```python
from build123d import *

# Parameters (mm, degrees)
SKETCH1_W           = 34
SKETCH1_H           = 70
BOSS_EXTRUDE1_DEPTH = 14
SKETCH2_W           = 30
SKETCH2_H           = 66
CUT_EXTRUDE1_DEPTH  = 12
SKETCH3_R           = 3
BOSS_EXTRUDE2_DEPTH = 12
SKETCH4_R           = 2
CUT_EXTRUDE2_DEPTH  = 80.069589603
CUT_EXTRUDE4_REACH  = 81.07
SKETCH6_R           = 2.5
SKETCH6_R_2         = 2
FILLET1_R           = 1
BOSS_EXTRUDE3_START = -8
SKETCH7_R           = 5
SKETCH7_R_2         = 3
BOSS_EXTRUDE3_DEPTH = 8
CUT_EXTRUDE7_START  = -4
SKETCH8_R           = 3
CUT_EXTRUDE7_DEPTH  = 4
FILLET2_R           = 2


with BuildPart() as part:
    # Sketch1 → Boss-Extrude1 (new body)
    with BuildSketch(Plane.XY):
        with Locations((17, 35)):
            Rectangle(SKETCH1_W, SKETCH1_H)
    extrude(amount=BOSS_EXTRUDE1_DEPTH)

    # Sketch2 → Cut-Extrude1 (cut)
    with BuildSketch(Plane(origin=(0, 0, 0), x_dir=(-1, 0, 0), z_dir=(0, 0, -1))):
        with Locations((-17, 35)):
            Rectangle(SKETCH2_W, SKETCH2_H)
    extrude(amount=-CUT_EXTRUDE1_DEPTH, mode=Mode.SUBTRACT)

    # Sketch3 → Boss-Extrude2 (add)
    with BuildSketch(Plane(origin=(0, 0, 0), x_dir=(-1, 0, 0), z_dir=(0, 0, -1))):
        with Locations((-31, 67)):
            Circle(SKETCH3_R)
        with Locations((-3, 67)):
            Circle(SKETCH3_R)
        with Locations((-3, 3)):
            Circle(SKETCH3_R)
        with Locations((-31, 3)):
            Circle(SKETCH3_R)
    extrude(amount=-BOSS_EXTRUDE2_DEPTH)

    # Sketch4 → Cut-Extrude2 (cut, through all)
    with BuildSketch(Plane(origin=(0, 0, 0), x_dir=(-1, 0, 0), z_dir=(0, 0, -1))):
        with Locations((-3, 67)):
            Circle(SKETCH4_R)
        with Locations((-31, 67)):
            Circle(SKETCH4_R)
        with Locations((-3, 3)):
            Circle(SKETCH4_R)
        with Locations((-31, 3)):
            Circle(SKETCH4_R)
    extrude(amount=-CUT_EXTRUDE2_DEPTH, mode=Mode.SUBTRACT)

    # Sketch6 → Cut-Extrude4 (cut, up to next)
    with BuildSketch(Plane.XZ, mode=Mode.PRIVATE) as cut_extrude4_sk1:
        with Locations((9.5, 0)):
            Circle(SKETCH6_R)
    cut_extrude4_tool1 = extrude(cut_extrude4_sk1.sketch, amount=-CUT_EXTRUDE4_REACH, mode=Mode.PRIVATE) & part.part
    # Sketch6 → Cut-Extrude4 (cut, up to next)
    with BuildSketch(Plane.XZ, mode=Mode.PRIVATE) as cut_extrude4_sk2:
        with Locations((24.5, 0)):
            Circle(SKETCH6_R_2)
    cut_extrude4_tool2 = extrude(cut_extrude4_sk2.sketch, amount=-CUT_EXTRUDE4_REACH, mode=Mode.PRIVATE) & part.part
    add(cut_extrude4_tool1.solids().sort_by_distance((9.5, 0, 0))[0], mode=Mode.SUBTRACT)
    add(cut_extrude4_tool2.solids().sort_by_distance((24.5, 0, 0))[0], mode=Mode.SUBTRACT)

    # Fillet1
    fillet1_edges = [part.edges().sort_by_distance(p)[0] for p in [
        (0, 70, 7),
        (34, 70, 7),
        (34, 0, 7),
        (0, 0, 7),
    ]]
    fillet(fillet1_edges, radius=FILLET1_R)

    # Sketch7 → Boss-Extrude3 (add)
    # profile 1 of 4: a face of its own
    with BuildSketch(Plane.XY.offset(14).offset(BOSS_EXTRUDE3_START)):
        with Locations((31, 67)):
            Circle(SKETCH7_R)
        with Locations((31, 67)):
            Circle(SKETCH7_R_2, mode=Mode.SUBTRACT)
    # profile 2 of 4: a face of its own
    with BuildSketch(Plane.XY.offset(14).offset(BOSS_EXTRUDE3_START)):
        with Locations((3, 67)):
            Circle(SKETCH7_R)
        with Locations((3, 67)):
            Circle(SKETCH7_R_2, mode=Mode.SUBTRACT)
    # profile 3 of 4: a face of its own
    with BuildSketch(Plane.XY.offset(14).offset(BOSS_EXTRUDE3_START)):
        with Locations((31, 3)):
            Circle(SKETCH7_R)
        with Locations((31, 3)):
            Circle(SKETCH7_R_2, mode=Mode.SUBTRACT)
    # profile 4 of 4: a face of its own
    with BuildSketch(Plane.XY.offset(14).offset(BOSS_EXTRUDE3_START)):
        with Locations((3, 3)):
            Circle(SKETCH7_R)
        with Locations((3, 3)):
            Circle(SKETCH7_R_2, mode=Mode.SUBTRACT)
    extrude(amount=BOSS_EXTRUDE3_DEPTH)

    # Sketch8 → Cut-Extrude7 (cut)
    with BuildSketch(Plane.XY.offset(14).offset(CUT_EXTRUDE7_START)):
        with Locations((3, 3)):
            Circle(SKETCH8_R)
        with Locations((31, 3)):
            Circle(SKETCH8_R)
        with Locations((31, 67)):
            Circle(SKETCH8_R)
        with Locations((3, 67)):
            Circle(SKETCH8_R)
    extrude(amount=CUT_EXTRUDE7_DEPTH, mode=Mode.SUBTRACT)

    # Fillet2
    # the kernel refuses this fillet: 2 mm, written as the material it adds along each edge
    with BuildSketch(Plane(origin=(3, 67, 10), x_dir=(1, 0, 0), z_dir=(0, -1, 0))) as fillet2_piece_1_section:
        with BuildLine():
            CenterArc((1, 1.732050808), FILLET2_R, 300, 60)
            Line((2, 0), (2.02, -0.034641016))
            ThreePointArc((2.02, -0.034641016), (2.5, -0.04), (3, -0.04))
            Line((3, -0.04), (3.04, 0))
            Line((3.04, 0), (3.04, 1.732050808))
            Line((3.04, 1.732050808), (3, 1.732050808))
        make_face()
    fillet2_piece_1 = revolve(axis=Axis((3, 67, 10), (0, 0, 1)), mode=Mode.PRIVATE)
    fillet2_piece_1 = fillet2_piece_1 - Plane(origin=(3, 67, 10.721085361), x_dir=(-1, 0, 0), z_dir=(0, 0, -1)) * Cylinder(2, 13, mode=Mode.PRIVATE)
    add(fillet2_piece_1)
    with BuildSketch(Plane(origin=(31, 67, 10), x_dir=(1, 0, 0), z_dir=(0, -1, 0))) as fillet2_piece_2_section:
        with BuildLine():
            CenterArc((1, 1.732050808), FILLET2_R, 300, 60)
            Line((2, 0), (2.02, -0.034641016))
            ThreePointArc((2.02, -0.034641016), (2.5, -0.04), (3, -0.04))
            Line((3, -0.04), (3.04, 0))
            Line((3.04, 0), (3.04, 1.732050808))
            Line((3.04, 1.732050808), (3, 1.732050808))
        make_face()
    fillet2_piece_2 = revolve(axis=Axis((31, 67, 10), (0, 0, 1)), mode=Mode.PRIVATE)
    fillet2_piece_2 = fillet2_piece_2 - Plane(origin=(31, 67, 10.721085361), x_dir=(-1, 0, 0), z_dir=(0, 0, -1)) * Cylinder(2, 13, mode=Mode.PRIVATE)
    add(fillet2_piece_2)
    with BuildSketch(Plane(origin=(31, 3, 10), x_dir=(1, 0, 0), z_dir=(0, -1, 0))) as fillet2_piece_3_section:
        with BuildLine():
            CenterArc((1, 1.732050808), FILLET2_R, 300, 60)
            Line((2, 0), (2.02, -0.034641016))
            ThreePointArc((2.02, -0.034641016), (2.5, -0.04), (3, -0.04))
            Line((3, -0.04), (3.04, 0))
            Line((3.04, 0), (3.04, 1.732050808))
            Line((3.04, 1.732050808), (3, 1.732050808))
        make_face()
    fillet2_piece_3 = revolve(axis=Axis((31, 3, 10), (0, 0, 1)), mode=Mode.PRIVATE)
    fillet2_piece_3 = fillet2_piece_3 - Plane(origin=(31, 3, 10.721085361), x_dir=(-1, 0, 0), z_dir=(0, 0, -1)) * Cylinder(2, 13, mode=Mode.PRIVATE)
    add(fillet2_piece_3)
    with BuildSketch(Plane(origin=(3, 3, 10), x_dir=(1, 0, 0), z_dir=(0, -1, 0))) as fillet2_piece_4_section:
        with BuildLine():
            CenterArc((1, 1.732050808), FILLET2_R, 300, 60)
            Line((2, 0), (2.02, -0.034641016))
            ThreePointArc((2.02, -0.034641016), (2.5, -0.04), (3, -0.04))
            Line((3, -0.04), (3.04, 0))
            Line((3.04, 0), (3.04, 1.732050808))
            Line((3.04, 1.732050808), (3, 1.732050808))
        make_face()
    fillet2_piece_4 = revolve(axis=Axis((3, 3, 10), (0, 0, 1)), mode=Mode.PRIVATE)
    fillet2_piece_4 = fillet2_piece_4 - Plane(origin=(3, 3, 10.721085361), x_dir=(-1, 0, 0), z_dir=(0, 0, -1)) * Cylinder(2, 13, mode=Mode.PRIVATE)
    add(fillet2_piece_4)


solid = part.part
```
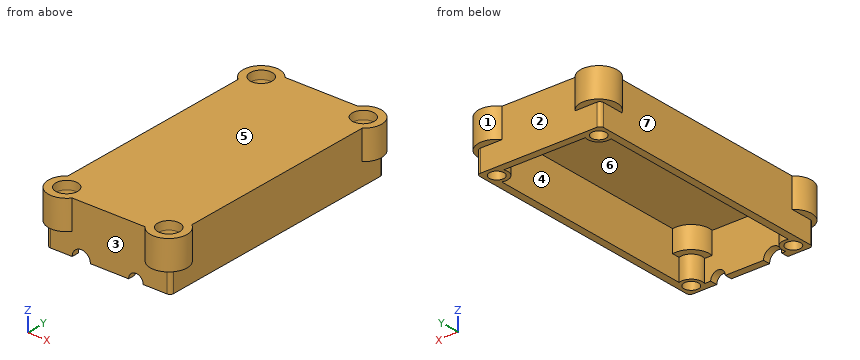
Design review of the part built by this model. Coordinates are the model's own, in mm. Face numbers are marked on the shaded views. A direction names the side the tool comes from. Give positions to 0.01 mm unless a question says otherwise; leave off trailing zeros. Order: outer loops, then holes, each group sorted by start corner. A loop starts at its lowest first (then second) coordinate and runs counter-clockwise, first axis right, second up. Notation, with made-up numbers: M 52,66.5 L 81,66.5 A30 ccw 81,95.5 Z; hole C 54,-19 d6. An arc over 180 degrees is marked long. One line per question, with ' | ' between items. Start each with the question number.
Q1. For L1, parallel to Y at x = 31, z = 7; L2, parallel to X at y = 67, z = 7.25; L3, parallel to X at y = 3, z = 4.5, list the stretches that pass through material, from the lowest coordinate up. Write a range as [from, to].
Q2. We need section C-C (x = 24.5). Write out the cut boundary in (y, z), plus the area to 3 significant figures.
Q3. We need section D-D (x = 31). State how many separate pieces and enclosed holes the cut face has, plus the area to 3 significant figures.
Q4. For pin 1 Ø1.5 at (x, z) = (26.5, 12.5) entering from -Y; pin 2 Ø4.5 at (x, y) = (31, 67) entering from +Z; pin 3 Ø6 at (x, z) = (21.5, 4) entering from +Y, all flat-tipped, find the tip position at first contact; note any pin that passes through.
Q5. We need section A-A (z = 3.25). Write out the cut boundary in (x, y).
Q6. Machinability: for the marked faces 1, 2, 3 and 4, which of the approach directions +Z, -Z, +X, -X, +Y, -Y give a long, thin tool a straight path to every point of the face, cutting with its end or side? Answer none if there is none.
Q7. We need section B-B (y = 58). Write out the cut boundary in (x, z).
Q8. The part is to be moulded in two halves that separate along X. For the marked faces 5, 6 and 7, say which applies: +X half, -X half, draft (parallel to the pull), parting line (faces both ways), or undercut.
Returned:
1) L1: [-2, 1], [5, 8], [62, 65], [69, 72] | L2: [-2, 1], [5, 8], [26, 29], [33, 36] | L3: [0, 1], [5, 6], [28, 29], [33, 34]
2) outline: M 0,2 L 2,2 L 2,12 L 68,12 L 68,0 L 70,0 L 70,14 L 0,14 Z | area: 184 mm2
3) separate pieces: 3 | enclosed holes: 0 | area: 214 mm2
4) pin 1: y = -0.31 | pin 2: z = 10.17 | pin 3: y = 70
5) outline: M 0,1 A1 ccw 1,0 L 33,0 A1 ccw 34,1 L 34,69 A1 ccw 33,70 L 1,70 A1 ccw 0,69 Z; hole C 3,3 d4; hole C 3,67 d4; hole M 2,5.83 A3 cw 5.83,2 L 28.17,2 A3 cw 32,5.83 L 32,64.17 A3 cw 28.17,68 L 5.83,68 A3 cw 2,64.17 Z; hole C 31,3 d4; hole C 31,67 d4
6) face 1: +Z, -Z | face 2: -Z, +Y | face 3: -Z, -Y | face 4: -Z
7) outline: M 0,0 L 2,0 L 2,12 L 32,12 L 32,0 L 34,0 L 34,14 L 0,14 Z
8) face 5: draft | face 6: undercut | face 7: -X half
